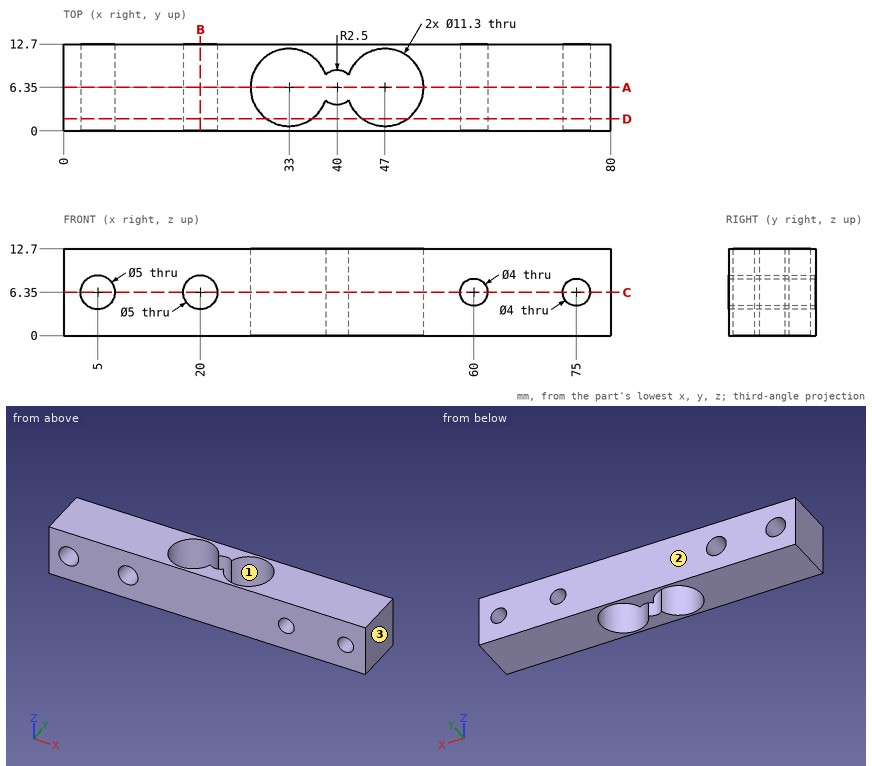
Design review of the part shown in the three views and the two pictorial views. Dimensions are in mm from the part's minimum x, y and z. Give positions to 0.01 mm unless a question says otherwise; leave off trailing zeros. Write each loop counter-clockwise with the first axis right and the second up, starting at its lowest first coordinate (ties: lowest second). Pieces come first, ordered by that corner, then holes. Notation, with made-up numbers: M -5,12 L 11,12 A21 cw 11,22 Z; hole C -31.75,61.5 d10. An arc over 180 degrees is marked long. Return JSON: item names as keys, results as strings. Group by question number.
Item 1: Take a section at C-C (z = 6.35). Give the boundary of the cut face in (x, y), plus the area to 3 significant figures.
Item 2: Take a section at A-A (y = 6.35). Give the boundary of the cut face in (x, z).
Item 3: Take a section at D-D (y = 1.75). Give the boundary of the cut face in (x, z), plus the area to 3 significant figures.
Item 4: Take a section at B-B (x = 20). Give the boundary of the cut face in (y, z).
Item 5: The part is to be moulded in two halves that separate along X. For the marked faces 1, 2 and 3, say which applies: pulls with the +X half, pulls with the -X half, needs draft (parallel to the pull), parting line crosses it, or undercut.
Item 6: Wall thickness on line 1 along Z through (x, y) = (75, 5.25); line 2 along Y through (x, z) = (40, 5.25); line 3 along X through (y, z) = (1.5, 2.75): over which ranges is each line inside the solid? List them lowest first.
Return value:
{
 "1": {"outline": "M 0,0 L 2.5,0 L 2.5,12.7 L 0,12.7 Z; M 7.5,0 L 17.5,0 L 17.5,12.7 L 7.5,12.7 Z; M 22.5,0 L 58,0 L 58,12.7 L 22.5,12.7 Z; M 62,0 L 73,0 L 73,12.7 L 62,12.7 Z; M 77,0 L 80,0 L 80,12.7 L 77,12.7 Z; hole M 38.33,4.49 A2.5 ccw 41.67,4.49 A5.65 ccw long 41.67,8.21 A2.5 ccw 38.33,8.21 A5.65 ccw long Z", "area": "573 mm2"},
 "2": {"outline": "M 0,0 L 27.35,0 L 27.35,12.7 L 0,12.7 Z; M 52.65,0 L 80,0 L 80,12.7 L 52.65,12.7 Z; hole C 5,6.35 d5; hole C 20,6.35 d5; hole C 60,6.35 d4; hole C 75,6.35 d4"},
 "3": {"outline": "M 0,0 L 29.72,0 L 29.72,12.7 L 0,12.7 Z; M 36.28,0 L 43.72,0 L 43.72,12.7 L 36.28,12.7 Z; M 50.28,0 L 80,0 L 80,12.7 L 50.28,12.7 Z; hole C 5,6.35 d5; hole C 20,6.35 d5; hole C 60,6.35 d4; hole C 75,6.35 d4", "area": "785 mm2"},
 "4": {"outline": "M 0,0 L 12.7,0 L 12.7,3.85 L 0,3.85 Z; M 0,8.85 L 12.7,8.85 L 12.7,12.7 L 0,12.7 Z"},
 "5": {"face 1": "undercut", "face 2": "needs draft", "face 3": "pulls with the +X half"},
 "6": {"line 1": "z = 0 to 4.35, 8.35 to 12.7", "line 2": "y = 0 to 3.85, 8.85 to 12.7", "line 3": "x = 0 to 30.1, 35.9 to 44.1, 49.9 to 80"}
}
